```python
from build123d import *

# Parameters (mm, degrees)
THICKNESS_MAINOUTLINE_DEPTH = 11.43
CORNERPOCKETRADIUS_R        = 3.302
CUT_EXTRUDE4_DEPTH          = 11.43
FLANGEDEPTH_DEPTH           = 3.175
SCREWHOLES_R                = 1.5875
CUT_EXTRUDE2_DEPTH          = 11.43
PLEXCHANNEL_W               = 363.5375
PLEXCHANNEL_H               = 6.35
PLEXCHANNEL_DEPTH_DEPTH     = 6.35
SKETCH7_W                   = 101.6
SKETCH7_H                   = 5.08
EXTRUDE2_DEPTH              = 11.43
SKETCH8_R                   = 3.175
CUT_EXTRUDE5_DEPTH          = 11.43


with BuildPart() as part:
    # MainOutline → Thickness_MainOutline (new body)
    with BuildSketch(Plane.XY):
        with BuildLine():
            Line((-5740.4, 1539.24), (-5740.4, 1384.3))
            Line((-5740.4, 1384.3), (-5584.03125, 1384.3))
            Line((-5584.03125, 1384.3), (-5584.03125, 1392.2375))
            ThreePointArc((-5584.03125, 1392.2375), (-5581.706410076, 1397.850160076), (-5576.09375, 1400.175))
            Line((-5576.09375, 1400.175), (-5506.24375, 1400.175))
            ThreePointArc((-5506.24375, 1400.175), (-5500.631089924, 1397.850160076), (-5498.30625, 1392.2375))
            Line((-5498.30625, 1392.2375), (-5498.30625, 1384.3))
            Line((-5498.30625, 1384.3), (-5451.475, 1384.3))
            Line((-5451.475, 1384.3), (-5451.475, 1512.8875))
            ThreePointArc((-5451.475, 1512.8875), (-5450.54506403, 1515.13256403), (-5448.3, 1516.0625))
            Line((-5448.3, 1516.0625), (-5303.8375, 1516.0625))
            ThreePointArc((-5303.8375, 1516.0625), (-5301.59243597, 1515.13256403), (-5300.6625, 1512.8875))
            Line((-5300.6625, 1512.8875), (-5300.6625, 1384.3))
            Line((-5300.6625, 1384.3), (-5253.83125, 1384.3))
            Line((-5253.83125, 1384.3), (-5253.83125, 1392.2375))
            ThreePointArc((-5253.83125, 1392.2375), (-5251.506410076, 1397.850160076), (-5245.89375, 1400.175))
            Line((-5245.89375, 1400.175), (-5176.04375, 1400.175))
            ThreePointArc((-5176.04375, 1400.175), (-5170.431089924, 1397.850160076), (-5168.10625, 1392.2375))
            Line((-5168.10625, 1392.2375), (-5168.10625, 1384.3))
            Line((-5168.10625, 1384.3), (-5011.7375, 1384.3))
            Line((-5011.7375, 1384.3), (-5011.7375, 1539.24))
            Line((-5011.7375, 1539.24), (-5194.3, 1539.24))
            Line((-5194.3, 1539.24), (-5194.3, 1550.67))
            Line((-5194.3, 1550.67), (-5557.8375, 1550.67))
            Line((-5557.8375, 1550.67), (-5557.8375, 1539.24))
            Line((-5557.8375, 1539.24), (-5740.4, 1539.24))
        make_face()
    extrude(amount=-THICKNESS_MAINOUTLINE_DEPTH)

    # CornerPocketRadius → Cut-Extrude4 (cut)
    with BuildSketch(Plane.XY):
        with Locations((-5560.08256403, 1541.48506403)):
            Circle(CORNERPOCKETRADIUS_R)
        with Locations((-5192.05493597, 1541.48506403)):
            Circle(CORNERPOCKETRADIUS_R)
    extrude(amount=-CUT_EXTRUDE4_DEPTH, mode=Mode.SUBTRACT)

    # PowerBoxFlange → FlangeDepth (cut)
    with BuildSketch(Plane.XY):
        with BuildLine():
            Line((-5297.4875, 1377.95), (-5454.65, 1377.95))
            ThreePointArc((-5454.65, 1377.95), (-5459.140128061, 1379.809871939), (-5461, 1384.3))
            Line((-5461, 1384.3), (-5461, 1516.0625))
            ThreePointArc((-5461, 1516.0625), (-5458.210192091, 1522.797692091), (-5451.475, 1525.5875))
            Line((-5451.475, 1525.5875), (-5300.6625, 1525.5875))
            ThreePointArc((-5300.6625, 1525.5875), (-5293.927307909, 1522.797692091), (-5291.1375, 1516.0625))
            Line((-5291.1375, 1516.0625), (-5291.1375, 1384.3))
            ThreePointArc((-5291.1375, 1384.3), (-5292.997371939, 1379.809871939), (-5297.4875, 1377.95))
        make_face()
    extrude(amount=-FLANGEDEPTH_DEPTH, mode=Mode.SUBTRACT)

    # ScrewHoles → Cut-Extrude2 (cut)
    with BuildSketch(Plane.XY):
        with Locations((-5734.05, 1511.3)):
            Circle(SCREWHOLES_R)
        with Locations((-5734.05, 1409.7)):
            Circle(SCREWHOLES_R)
        with Locations((-5018.0875, 1409.7)):
            Circle(SCREWHOLES_R)
        with Locations((-5018.0875, 1511.3)):
            Circle(SCREWHOLES_R)
    extrude(amount=-CUT_EXTRUDE2_DEPTH, mode=Mode.SUBTRACT)

    # PlexChannel → PlexChannel_Depth (cut)
    with BuildSketch(Plane(origin=(0, 0, -11.43), x_dir=(-1, 0, 0), z_dir=(0, 0, -1))):
        with Locations((5376.06875, 1543.05)):
            Rectangle(PLEXCHANNEL_W, PLEXCHANNEL_H)
    extrude(amount=-PLEXCHANNEL_DEPTH_DEPTH, mode=Mode.SUBTRACT)

    # Sketch7 → Extrude2 (add)
    with BuildSketch(Plane.XY):
        with Locations((-5689.6, 1381.76)):
            Rectangle(SKETCH7_W, SKETCH7_H)
        with Locations((-5062.5375, 1381.76)):
            Rectangle(SKETCH7_W, SKETCH7_H)
    extrude(amount=-EXTRUDE2_DEPTH)

    # Sketch8 → Cut-Extrude5 (cut)
    with BuildSketch(Plane.XY):
        with Locations((-5635.625, 1384.3)):
            Circle(SKETCH8_R)
        with Locations((-5116.5125, 1384.3)):
            Circle(SKETCH8_R)
    extrude(amount=-CUT_EXTRUDE5_DEPTH, mode=Mode.SUBTRACT)


solid = part.part
```
CAD build for the part. Positions are in the model's coordinates, mm. A direction names the side the tool comes from. Coordinates: 2 decimals unless noted, no trailing zeros. Order: outer loops, then holes, each group sorted by start corner. A loop starts at its lowest first (then second) coordinate and runs counter-clockwise, first axis right, second up.
(1) Saw through at A-A, the plane y = 1473. Write the cut outline in (x, z) (1 decimal), and give its area (3 significant figures).
Solution:
outline: (-5740.4, -11.4) - (-5451.5, -11.4) - (-5451.5, -3.2) - (-5461, -3.2) - (-5461, 0) - (-5740.4, 0) - close; (-5300.7, -11.4) - (-5011.7, -11.4) - (-5011.7, 0) - (-5291.1, 0) - (-5291.1, -3.2) - (-5300.7, -3.2) - close
area: 6,540 mm2
(2) Mould opens along X. For faces 1 (the face through (-5363, 1518, -3.175)), 2 (the face through (-5650, 1539.24, -6)), 3 (the face through (-5011.738, 1458, -6)) say: released by +X, released by -X, zero draft, split by the parting line, or undercut.
Solution:
face 1: undercut
face 2: zero draft
face 3: released by +X
(3) Which spindle directions (+Z, -Z, +X, -X, +Y, -Y) get a long thin tool onto all of the face, cutting with end or side? Do faces 4 (the face through (-5374, 1550.67, -6)), 5 (the face through (-5099, 1539.24, -6)), 6 (the face through (-5211, 1400.175, -6)). Say none if no direction does.
Solution:
face 4: +Z, -Z, +X, -X, +Y
face 5: +Z, -Z, +X, +Y
face 6: +Z, -Z, -Y
(4) Saw through at B-B, the plane z = -7.25. Count the separate pieces of the cut face and the enclosed holes in it, and give its area (3 significant figures).
Solution:
separate pieces: 2
enclosed holes: 4
area: 93,200 mm2
(5) Drill centre lines: L1, parallel to X at y = 1511.3, z = -6.75 (1 decimal); L2, parallel to X at y = 1511.3, z = -2.25 (1 decimal); L3, parallel to Y at x = -5734.05, z = -9. Where is each one in solid material? Low to high.
Solution:
L1: x = -5740.4 to -5735.6, -5732.5 to -5451.5, -5300.7 to -5019.7, -5016.5 to -5011.7
L2: x = -5740.4 to -5735.6, -5732.5 to -5461, -5291.1 to -5019.7, -5016.5 to -5011.7
L3: y = 1379.22 to 1408.11, 1411.29 to 1509.71, 1512.89 to 1539.24
(6) Pin check, flat tips, straight feed: pin 1 Ø2 at (x, y) = (-5567.5, 1498.5) entering from +Z; pin 2 Ø5.5 at (x, z) = (-5135, -3) entering from -Y; pin 3 Ø3.5 at (x, z) = (-5382, -2) entering from -Y; pin 4 Ø2.5 at (x, y) = (-5734.05, 1511.3) entering from +Z. Stop position of each tip, or through.
Solution:
pin 1: stops at z = 0
pin 2: stops at y = 1384.3
pin 3: stops at y = 1516.06
pin 4: passes through
(7) Saw through at D-D, the plane x = -5470.5. Write the cut outline in (y, z) (3 decimals).
Solution:
outline: (1384.3, -11.43) - (1539.875, -11.43) - (1539.875, -5.08) - (1546.225, -5.08) - (1546.225, -11.43) - (1550.67, -11.43) - (1550.67, 0) - (1384.3, 0) - close
(8) Saw through at C-C, the plane x = -5383.5. Write the cut outline in (y, z) (1 decimal), and give its area (3 significant figures).
Solution:
outline: (1516.1, -11.4) - (1539.9, -11.4) - (1539.9, -5.1) - (1546.2, -5.1) - (1546.2, -11.4) - (1550.7, -11.4) - (1550.7, 0) - (1525.6, 0) - (1525.6, -3.2) - (1516.1, -3.2) - close
area: 325 mm2
